from build123d import *

# Parameters (mm, degrees)
F0_W      = 310
F0_H      = 220
F1_DEPTH  = 40
F2_T      = -15
F4_D      = 10
F4_DEPTH  = 15
F4_TIP    = 3.0043030951
F6_D      = 3
F6_DEPTH  = 10
F6_TIP    = 0.9012909285
F7_DEPTH  = 20
F9_D      = 7
F9_DEPTH  = 100
F9_TIP    = 2.1030121666
F11_D     = 7
F11_DEPTH = 100
F11_TIP   = 2.1030121666
F12_W     = 286
F12_H     = 2
F13_DEPTH = 2


with BuildPart() as f1:
    # F0 (on Front) → F1 (new body)
    with BuildSketch(Plane.XZ):
        Rectangle(F0_W, F0_H)
    extrude(amount=F1_DEPTH)

    # F2
    f2_openings = [f1.faces().sort_by_distance(p)[0] for p in [
        (0, -40, 0),
    ]]
    offset(amount=F2_T, openings=f2_openings)

    # F4
    with Locations(Plane.YZ.offset(155)):
        with Locations((-25, -55), (-25, 55)):
            Hole(F4_D / 2, depth=F4_DEPTH)
            with Locations((0, 0, -(F4_DEPTH + F4_TIP / 2))):  # 118° drill point
                Cone(0, F4_D / 2, F4_TIP, mode=Mode.SUBTRACT)

    # F6
    with Locations(Plane.XZ.offset(40)):
        with Locations((-150, -105), (-150, 0), (-150, 105), (-75, 105), (-75, -105), (0, -105), (75, -105), (150, -105), (150, 0), (150, 105), (75, 105), (0, 105)):
            Hole(F6_D / 2, depth=F6_DEPTH)
            with Locations((0, 0, -(F6_DEPTH + F6_TIP / 2))):  # 118° drill point
                Cone(0, F6_D / 2, F6_TIP, mode=Mode.SUBTRACT)

    # F7 (add): a face of the model
    f7_faces = [f1.faces().sort_by_distance(p)[0] for p in [
        (0, 0, 0),
    ]]
    extrude(f7_faces, amount=F7_DEPTH)

    # F9
    with Locations(Plane(origin=(-155, 0, 0), x_dir=(0, -1, 0), z_dir=(-1, 0, 0))):
        with Locations((-10, 80), (-10, 0), (-10, -80)):
            Hole(F9_D / 2, depth=F9_DEPTH)
            with Locations((0, 0, -(F9_DEPTH + F9_TIP / 2))):  # 118° drill point
                Cone(0, F9_D / 2, F9_TIP, mode=Mode.SUBTRACT)

    # F11
    with Locations(Plane.YZ.offset(155)):
        with Locations((10, -80), (10, 0), (10, 80)):
            Hole(F11_D / 2, depth=F11_DEPTH)
            with Locations((0, 0, -(F11_DEPTH + F11_TIP / 2))):  # 118° drill point
                Cone(0, F11_D / 2, F11_TIP, mode=Mode.SUBTRACT)

    # F12 (on face) → F13 (cut)
    with BuildSketch(Plane.XZ.offset(40)):
        Polygon((-145, -100), (-143, -100), (-143, -98), (-143, 98), (-143, 100), (-145, 100), align=None)
        with Locations((0, -99)):
            Rectangle(F12_W, F12_H)
        Polygon((143, -98), (143, -100), (145, -100), (145, 100), (143, 100), (143, 98), align=None)
        with Locations((0, 99)):
            Rectangle(F12_W, F12_H)
    extrude(amount=-F13_DEPTH, mode=Mode.SUBTRACT)


solid = f1.part
The model under review builds one solid part; all positions refer to its coordinate system, in mm. A direction names the side the tool comes from. Round coordinates to 2 decimals unless told otherwise and drop trailing zeros. Loops run counter-clockwise (first coordinate to the right, second up) from the corner with the lowest first, then second, coordinate; pieces in that order, holes last. Notation, with made-up numbers: M -36.5,-29.75 L -5.5,-29.75 A22 cw -5.5,3.25 Z; hole C 36.5,83 d8. An arc over 180 degrees is marked long. Answer as CSV lines item,"result".
1. Insertion check: pin 1 Ø3.5 at (x, z) = (-150, 105) entering from -Y; pin 2 Ø3 at (x, z) = (10.5, -77.5) entering from -Y; pin 3 Ø1.8 at (x, z) = (0, 105) entering from -Y. Each pin has a flat end and moves straight along its axis. Give the tip position at first contact, or say it passes through.
Outcome:
pin 1,"stops at y = -40"
pin 2,"stops at y = -15"
pin 3,"stops at y = -29.64"
2. We need section B-B (z = -39). Give the boundary of the cut face in (x, y), plus the area to 3 significant figures.
Outcome:
outline,"M -155,-40 L -145,-40 L -145,-38 L -143,-38 L -143,-40 L -140,-40 L -140,-15 L 140,-15 L 140,-40 L 143,-40 L 143,-38 L 145,-38 L 145,-40 L 155,-40 L 155,20 L -155,20 Z"
area,"11,600 mm2"
3. We need section A-A (x = 61.5). Give the boundary of the cut face in (y, z).
Outcome:
outline,"M -40,-110 L 20,-110 L 20,110 L -40,110 L -40,100 L -38,100 L -38,98 L -40,98 L -40,95 L -15,95 L -15,-95 L -40,-95 L -40,-98 L -38,-98 L -38,-100 L -40,-100 Z; hole C 10,-80 d7; hole C 10,0 d7; hole C 10,80 d7"
4. To check wall thickness, follow L1, parallel to Z at x = 150, y = -34; L2, parallel to X at y = -33.75, z = 105; L3, parallel to Z at x = -101, y = 10. State the ranges of each line that lie inside material, in increasing order. Write a range as [from, to].
Outcome:
L1,"z = [-110, -106.5], [-103.5, -1.5], [1.5, 103.5], [106.5, 110]"
L2,"x = [-155, -151.5], [-148.5, -76.5], [-73.5, -1.5], [1.5, 73.5], [76.5, 148.5], [151.5, 155]"
L3,"z = [-110, -83.5], [-76.5, -3.5], [3.5, 76.5], [83.5, 110]"
5. For faces 1 (the face through (-2, -27, 95)), 2 (the face through (-2, -10, -110)), 3 (the face through (147.395, -24.349, -50.043)), list the 3-axis set-ups (+Z, -Z, +X, -X, +Y, -Y) from which the entire face can be reached by the end or side of a thin tool; tool diameter is ignored.
Outcome:
face 1,"-Y"
face 2,"-Z, +X, -X, +Y, -Y"
face 3,"+X"
6. Draft analysis for pull direction Y (two halves, no side actions). For faces 4 (the face through (-2, 20, 2)), 5 (the face through (-53.26, 10.08, 80.6)), 6 (the face through (-2, -15, 1)), state which applies: pulls with the +Y half, pulls with the -Y half, needs draft (parallel to the pull), parting line crosses it, or undercut.
Outcome:
face 4,"pulls with the +Y half"
face 5,"undercut"
face 6,"pulls with the -Y half"
